The listing builds one solid part. Answer for the finished solid, in the listing's coordinates (mm). Coordinates: 2 decimals unless noted, no trailing zeros. Order: outer loops, then holes, each group sorted by start corner. A loop starts at its lowest first (then second) coordinate and runs counter-clockwise, first axis right, second up. Notation, with made-up numbers: (47.5, 15.25) -> (55.5, 15.25) arc R35 cw to (55.5, 52.25) -> close; hole circle Ø1 at (14.5, 71.25). An arc over 180 degrees is marked (long way). One line per question, with ' | ' between items.
from build123d import *

# Parameters (mm, degrees)
ESQUISSE1_W             = 200
ESQUISSE1_H             = 122
BOSS_EXTRU_1_DEPTH      = 6
ESQUISSE2_W             = 67
ESQUISSE2_H             = 6
ESQUISSE2_W_2           = 6
ESQUISSE2_H_2           = 30
ESQUISSE2_W_3           = 84
ESQUISSE2_H_3           = 42
ENL_V_MAT_EXTRU_1_DEPTH = 6
CONG_1_R                = 10
ESQUISSE3_R             = 1.5
ENL_V_MAT_EXTRU_2_DEPTH = 6
ESQUISSE4_R             = 2.995
ENL_V_MAT_EXTRU_3_DEPTH = 3


with BuildPart() as part:
    # Esquisse1 → Boss.-Extru.1 (new body)
    with BuildSketch(Plane.XY):
        with Locations((3.313253012, -9.644578313)):
            Rectangle(ESQUISSE1_W, ESQUISSE1_H)
    extrude(amount=BOSS_EXTRU_1_DEPTH)

    # Esquisse2 → Enlèv. mat.-Extru.1 (cut)
    with BuildSketch(Plane.XY.offset(6)):
        with Locations((3.313253012, 48.355421687)):
            Rectangle(ESQUISSE2_W, ESQUISSE2_H)
        with Locations((-93.686746988, 8.355421687)):
            Rectangle(ESQUISSE2_W_2, ESQUISSE2_H_2)
        with Locations((100.313253012, 8.355421687)):
            Rectangle(ESQUISSE2_W_2, ESQUISSE2_H_2)
        with Locations((3.313253012, -49.644578313)):
            Rectangle(ESQUISSE2_W_3, ESQUISSE2_H_3)
    extrude(amount=-ENL_V_MAT_EXTRU_1_DEPTH, mode=Mode.SUBTRACT)

    # Congé1
    cong_1_edges = [part.edges().sort_by_distance(p)[0] for p in [
        (-38.686746988, -28.644578313, 3),
        (45.313253012, -28.644578313, 3),
    ]]
    fillet(cong_1_edges, radius=CONG_1_R)

    # Esquisse3 → Enlèv. mat.-Extru.2 (cut)
    with BuildSketch(Plane.XY.offset(6)):
        with Locations((-93.686746988, -50.644578313)):
            Circle(ESQUISSE3_R)
        with Locations((-93.686746988, -26.644578313)):
            Circle(ESQUISSE3_R)
        with Locations((-93.686746988, 37.355421687)):
            Circle(ESQUISSE3_R)
        with Locations((-50.186746988, 48.355421687)):
            Circle(ESQUISSE3_R)
        with Locations((56.813253012, 48.355421687)):
            Circle(ESQUISSE3_R)
        with Locations((100.313253012, 37.355421687)):
            Circle(ESQUISSE3_R)
        with Locations((100.313253012, -26.644578313)):
            Circle(ESQUISSE3_R)
        with Locations((100.313253012, -50.644578313)):
            Circle(ESQUISSE3_R)
        with Locations((-82.686746988, 48.355421687)):
            Circle(ESQUISSE3_R)
        with Locations((89.313253012, 48.355421687)):
            Circle(ESQUISSE3_R)
    extrude(amount=-ENL_V_MAT_EXTRU_2_DEPTH, mode=Mode.SUBTRACT)

    # Esquisse4 → Enlèv. mat.-Extru.3 (cut)
    with BuildSketch(Plane.XY.offset(6)):
        with Locations((-93.686746988, -50.644578313)):
            Circle(ESQUISSE4_R)
        with Locations((-93.686746988, -26.644578313)):
            Circle(ESQUISSE4_R)
        with Locations((-93.686746988, 37.355421687)):
            Circle(ESQUISSE4_R)
        with Locations((-82.686746988, 48.355421687)):
            Circle(ESQUISSE4_R)
        with Locations((-50.186746988, 48.355421687)):
            Circle(ESQUISSE4_R)
        with Locations((56.813253012, 48.355421687)):
            Circle(ESQUISSE4_R)
        with Locations((89.313253012, 48.355421687)):
            Circle(ESQUISSE4_R)
        with Locations((100.313253012, 37.355421687)):
            Circle(ESQUISSE4_R)
        with Locations((100.313253012, -26.644578313)):
            Circle(ESQUISSE4_R)
        with Locations((100.313253012, -50.644578313)):
            Circle(ESQUISSE4_R)
    extrude(amount=-ENL_V_MAT_EXTRU_3_DEPTH, mode=Mode.SUBTRACT)


solid = part.part
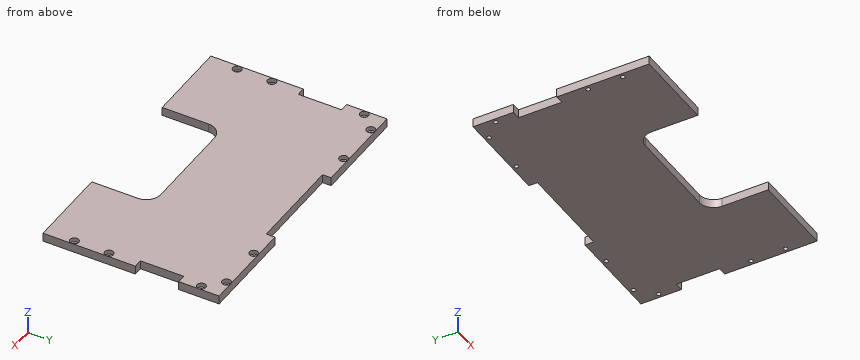
Item 1: Each of these flat-tipped pins is pushed along its axis until it touches: pin 1 Ø2.5 at (x, y) = (56.81, 48.36) entering from -Z; pin 2 Ø3 at (x, y) = (-95, -50) entering from +Z; pin 3 Ø2 at (x, z) = (26, 1) entering from -Y. Where does it stop, or does it pass through?
Computed values:
pin 1: passes through | pin 2: stops at z = 3 | pin 3: stops at y = -28.64
Item 2: Section A-A, the plane y = -42.5 is taken. Give the vertices of the cut face in (x, z).
Computed values:
outline: (-96.69, 0) -> (-38.69, 0) -> (-38.69, 6) -> (-96.69, 6) -> close; (45.31, 0) -> (103.31, 0) -> (103.31, 6) -> (45.31, 6) -> close
Item 3: Section D-D, the plane y = 9 is taken. Give the vertices of the cut face in (x, z).
Computed values:
outline: (-90.69, 0) -> (97.31, 0) -> (97.31, 6) -> (-90.69, 6) -> close
Item 4: Section C-C, the plane x = -33.5 is taken. Give the vertices of the cut face in (y, z), plus the area to 3 significant figures.
Computed values:
outline: (-29.88, 0) -> (51.36, 0) -> (51.36, 6) -> (-29.88, 6) -> close | area: 487 mm^2
Item 5: Find the intervals of material crossed by L1, parallel to X at y = -27, z = 1.3; L2, parallel to X at y = -40.5, z = 1.9; L3, parallel to X at y = 10, z = 5.55, in increasing order.
Computed values:
L1: x = -96.69 to -95.14, -92.23 to 98.86, 101.77 to 103.31 | L2: x = -96.69 to -38.69, 45.31 to 103.31 | L3: x = -90.69 to 97.31
Item 6: Section B-B, the plane z = 4.1 is taken. Count the separate pieces of the cut face and the enclosed holes in it, plus the area to 3 significant figures.
Computed values:
separate pieces: 1 | enclosed holes: 10 | area: 19,900 mm^2
